Could you check a few things on this model? Use its own coordinates, in mm. A direction names the side the tool comes from. Coordinates: 2 decimals unless noted, no trailing zeros. Loops run counter-clockwise (first coordinate to the right, second up) from the corner with the lowest first, then second, coordinate; pieces in that order, holes last. Notation, with made-up numbers: (14, 10) - (37, 10) arc R15 ccw to (37, 39) - close; hole circle Ø3 at (-21, 8). An arc over 180 degrees is marked (long way). One line per question, with ' | ' between items. Start each with the question number.
1. I want a section at D-D, the plane x = 22.5. Write out the boundary of the cut face in (y, z), then the cut area to 3 significant figures.
2. Which directions (+Z, -Z, +X, -X, +Y, -Y) give clear straight access to the entire face, cutting with the end or side of a thin tool? Please do faces 1 (the flat face through (-10, 0, 2)), 2 (the flat face through (60, 14, 1)), 3 (the flat face through (0, 7, 1)), 4 (the cylindrical face through (45.9, 71.64, 1.48)).
3. I'm going to push flat-ended pins straight in: P1, Ø10, axis at x = 36, y = 87.5, coming from the -Z side; P2, Ø3.5, axis at x = -10.5, z = 2, coming from the +Y side; P3, Ø4, axis at x = 43, z = 10, coming from the +Y side; P4, Ø1.5, axis at x = -29, y = 18.5, coming from the +Z side. Where does each tip first touch, or does it pass through?
4. I want a section at A-A, the plane z = 9.5. Count the separate pieces of the cut face and the enclosed holes in it, then the cut area to 3 significant figures.
5. I want a section at C-C, the plane y = 90. Write out the boundary of the cut face in (x, z), then the cut area to 3 significant figures.
6. We'd pull the mould along X, two halves only. Please class faces 5 (the cylindrical face through (0.86, 109.1, 1.52)), 6 (the flat face through (-31, 19, 18)), 7 (the cylindrical face through (-30.8, 20.27, 10.4)): pulls with the +X half, pulls with the -X half, needs draft (parallel to the pull), parting line crosses it, or undercut.
7. I want a section at B-B, the plane x = -10. Write out the boundary of the cut face in (y, z).
8. Please list where these lines run through material, in increasing order: L1, parallel to Y at x = -17, z = 3.6; L2, parallel to X at y = 101, z = 8.25; L3, parallel to X at y = 90, z = 1.3. Write a range as [from, to].
from build123d import *

# Parameters (mm, degrees)
SKETCH_1_W          = 60
SKETCH_1_H          = 100
EXTRUDE_1_DEPTH     = 3
CUT_EXTRUDE_1_REACH = 118.658
SKETCH_2_R          = 1.6
SKETCH_3_W          = 100
SKETCH_3_H          = 25
EXTRUDE_2_DEPTH     = 3
SKETCH_4_R          = 2.5
EXTRUDE_3_DEPTH     = 3
SKETCH_5_R          = 1
CUT_EXTRUDE_2_DEPTH = 129.202964084
SKETCH_6_W          = 45
SKETCH_6_H          = 5
EXTRUDE_4_DEPTH     = 5
SKETCH_7_W          = 75
SKETCH_7_H          = 5
EXTRUDE_5_DEPTH     = 5
SKETCH_8_R          = 0.6
CUT_EXTRUDE_3_DEPTH = 5
SKETCH_9_W          = 35
SKETCH_9_H          = 73
EXTRUDE_6_DEPTH     = 3
SKETCH_10_R         = 2.5
EXTRUDE_7_DEPTH     = 15
SKETCH_11_R         = 1.5
CUT_EXTRUDE_4_DEPTH = 10
SKETCH_12_W         = 60
SKETCH_12_H         = 10
EXTRUDE_8_DEPTH     = 28
CUT_EXTRUDE_5_REACH = 153.026
CUT_EXTRUDE_6_REACH = 160.458
SKETCH_14_R         = 1.5
CUT_EXTRUDE_7_REACH = 139.335
SKETCH_15_W         = 50
SKETCH_15_H         = 45
SKETCH_15_W_2       = 15
FILLET_1_R          = 3
FILLET_2_R          = 3
FILLET_3_R          = 3
FILLET_4_R          = 3
FILLET_5_R          = 3
FILLET_6_R          = 3


with BuildPart() as part:
    # 草图1 → 凸台-拉伸1 (new body)
    with BuildSketch(Plane.XY):
        with Locations((30, 50)):
            Rectangle(SKETCH_1_W, SKETCH_1_H)
    extrude(amount=EXTRUDE_1_DEPTH)

    # 草图2 → 切除-拉伸1 (cut, up to next)
    with BuildSketch(Plane.XY.offset(3), mode=Mode.PRIVATE) as cut_extrude_1_sk1:
        with Locations((7.5, 90)):
            Circle(SKETCH_2_R)
    cut_extrude_1_tool1 = extrude(cut_extrude_1_sk1.sketch, amount=-CUT_EXTRUDE_1_REACH, mode=Mode.PRIVATE) & part.part
    # 草图2 → 切除-拉伸1 (cut, up to next)
    with BuildSketch(Plane.XY.offset(3), mode=Mode.PRIVATE) as cut_extrude_1_sk2:
        with Locations((52.5, 90)):
            Circle(SKETCH_2_R)
    cut_extrude_1_tool2 = extrude(cut_extrude_1_sk2.sketch, amount=-CUT_EXTRUDE_1_REACH, mode=Mode.PRIVATE) & part.part
    # 草图2 → 切除-拉伸1 (cut, up to next)
    with BuildSketch(Plane.XY.offset(3), mode=Mode.PRIVATE) as cut_extrude_1_sk3:
        with Locations((52.5, 20)):
            Circle(SKETCH_2_R)
    cut_extrude_1_tool3 = extrude(cut_extrude_1_sk3.sketch, amount=-CUT_EXTRUDE_1_REACH, mode=Mode.PRIVATE) & part.part
    # 草图2 → 切除-拉伸1 (cut, up to next)
    with BuildSketch(Plane.XY.offset(3), mode=Mode.PRIVATE) as cut_extrude_1_sk4:
        with Locations((7.5, 20)):
            Circle(SKETCH_2_R)
    cut_extrude_1_tool4 = extrude(cut_extrude_1_sk4.sketch, amount=-CUT_EXTRUDE_1_REACH, mode=Mode.PRIVATE) & part.part
    add(cut_extrude_1_tool1.solids().sort_by_distance((7.5, 90, 3))[0], mode=Mode.SUBTRACT)
    add(cut_extrude_1_tool2.solids().sort_by_distance((52.5, 90, 3))[0], mode=Mode.SUBTRACT)
    add(cut_extrude_1_tool3.solids().sort_by_distance((52.5, 20, 3))[0], mode=Mode.SUBTRACT)
    add(cut_extrude_1_tool4.solids().sort_by_distance((7.5, 20, 3))[0], mode=Mode.SUBTRACT)

    # 草图3 → 凸台-拉伸2 (add)
    with BuildSketch(Plane.XY.offset(3)):
        with Locations((30, -12.5)):
            Rectangle(SKETCH_3_W, SKETCH_3_H)
    extrude(amount=-EXTRUDE_2_DEPTH)

    # 草图4 → 凸台-拉伸3 (add)
    with BuildSketch(Plane.XY.offset(3)):
        with Locations(Location((-17, -3.5, 0), (0, 0, 180))):
            Circle(SKETCH_4_R)
        with Locations(Location((-17, -21.5, 0), (0, 0, 180))):
            Circle(SKETCH_4_R)
        with Locations(Location((77, -21.5, 0), (0, 0, 180))):
            Circle(SKETCH_4_R)
        with Locations(Location((77, -3.5, 0), (0, 0, 180))):
            Circle(SKETCH_4_R)
    extrude(amount=EXTRUDE_3_DEPTH)

    # 草图5 → 切除-拉伸2 (cut, through all)
    with BuildSketch(Plane.XY.offset(6)):
        with Locations((-17, -3.5)):
            Circle(SKETCH_5_R)
        with Locations((-17, -21.5)):
            Circle(SKETCH_5_R)
        with Locations((77, -21.5)):
            Circle(SKETCH_5_R)
        with Locations((77, -3.5)):
            Circle(SKETCH_5_R)
    extrude(amount=-CUT_EXTRUDE_2_DEPTH, mode=Mode.SUBTRACT)

    # 草图6 → 凸台-拉伸4 (add)
    with BuildSketch(Plane.XY.offset(3)):
        with Locations((30, 7.5)):
            Rectangle(SKETCH_6_W, SKETCH_6_H)
    extrude(amount=EXTRUDE_4_DEPTH)

    # 草图7 → 凸台-拉伸5 (add)
    with BuildSketch(Plane.XY.offset(8)):
        with Locations((30, 7.5)):
            Rectangle(SKETCH_7_W, SKETCH_7_H)
    extrude(amount=EXTRUDE_5_DEPTH)

    # 草图8 → 切除-拉伸3 (cut)
    with BuildSketch(Plane.XY.offset(13)):
        with Locations((-5, 7.5)):
            Circle(SKETCH_8_R)
        with Locations((30, 7.5)):
            Circle(SKETCH_8_R)
        with Locations((65, 7.5)):
            Circle(SKETCH_8_R)
    extrude(amount=-CUT_EXTRUDE_3_DEPTH, mode=Mode.SUBTRACT)

    # 草图9 → 凸台-拉伸6 (add)
    with BuildSketch(Plane.XY.offset(3)):
        with Locations((-17.5, 50)):
            Rectangle(SKETCH_9_W, SKETCH_9_H)
    extrude(amount=-EXTRUDE_6_DEPTH)

    # 草图10 → 凸台-拉伸7 (add)
    with BuildSketch(Plane.XY.offset(3)):
        with Locations(Location((-29.65, 81.95, 0), (0, 0, 180))):
            Circle(SKETCH_10_R)
        with Locations(Location((-5.35, 81.95, 0), (0, 0, 180))):
            Circle(SKETCH_10_R)
        with Locations(Location((-5.35, 18.05, 0), (0, 0, 180))):
            Circle(SKETCH_10_R)
        with Locations(Location((-29.65, 18.05, 0), (0, 0, 180))):
            Circle(SKETCH_10_R)
    extrude(amount=EXTRUDE_7_DEPTH)

    # 草图11 → 切除-拉伸4 (cut)
    with BuildSketch(Plane.XY.offset(18)):
        with Locations((-29.65, 81.95)):
            Circle(SKETCH_11_R)
        with Locations((-5.35, 81.95)):
            Circle(SKETCH_11_R)
        with Locations((-5.35, 18.05)):
            Circle(SKETCH_11_R)
        with Locations((-29.65, 18.05)):
            Circle(SKETCH_11_R)
    extrude(amount=-CUT_EXTRUDE_4_DEPTH, mode=Mode.SUBTRACT)

    # 草图12 → 凸台-拉伸8 (add)
    with BuildSketch(Plane(origin=(0, 0, 0), x_dir=(-1, 0, 0), z_dir=(0, 0, -1))):
        with Locations((-30, 105)):
            Rectangle(SKETCH_12_W, SKETCH_12_H)
    extrude(amount=-EXTRUDE_8_DEPTH)

    # 草图13 → 切除-拉伸5 (cut, up to next)
    with BuildSketch(Plane.XZ.offset(-100), mode=Mode.PRIVATE) as cut_extrude_5_sk1:
        with BuildLine():
            Line((3.5, 3), (3.5, 18))
            ThreePointArc((3.5, 18), (7.5, 22), (11.5, 18))
            Line((11.5, 18), (11.5, 3))
            Line((11.5, 3), (48.5, 3))
            Line((48.5, 3), (48.5, 18))
            ThreePointArc((48.5, 18), (52.5, 22), (56.5, 18))
            Line((56.5, 18), (56.5, 3))
            Line((56.5, 3), (60, 3))
            Line((60, 3), (60, 28))
            Line((60, 28), (0, 28))
            Line((0, 28), (0, 3))
            Line((0, 3), (3.5, 3))
        make_face()
    cut_extrude_5_tool1 = extrude(cut_extrude_5_sk1.sketch, amount=-CUT_EXTRUDE_5_REACH, mode=Mode.PRIVATE) & part.part
    add(cut_extrude_5_tool1.solids().sort_by_distance((30, 100, 16.317537))[0], mode=Mode.SUBTRACT)

    # 草图14 → 切除-拉伸6 (cut, up to next)
    with BuildSketch(Plane(origin=(0, 110, 0), x_dir=(1, 0, 0), z_dir=(0, 1, 0)), mode=Mode.PRIVATE) as cut_extrude_6_sk1:
        with Locations(Location((7.5, -18, 0), (0, 0, 180))):
            Circle(SKETCH_14_R)
    cut_extrude_6_tool1 = extrude(cut_extrude_6_sk1.sketch, amount=-CUT_EXTRUDE_6_REACH, mode=Mode.PRIVATE) & part.part
    # 草图14 → 切除-拉伸6 (cut, up to next)
    with BuildSketch(Plane(origin=(0, 110, 0), x_dir=(1, 0, 0), z_dir=(0, 1, 0)), mode=Mode.PRIVATE) as cut_extrude_6_sk2:
        with Locations(Location((52.5, -18, 0), (0, 0, 180))):
            Circle(SKETCH_14_R)
    cut_extrude_6_tool2 = extrude(cut_extrude_6_sk2.sketch, amount=-CUT_EXTRUDE_6_REACH, mode=Mode.PRIVATE) & part.part
    add(cut_extrude_6_tool1.solids().sort_by_distance((7.5, 110, 18))[0], mode=Mode.SUBTRACT)
    add(cut_extrude_6_tool2.solids().sort_by_distance((52.5, 110, 18))[0], mode=Mode.SUBTRACT)

    # 草图15 → 切除-拉伸7 (cut, up to next)
    with BuildSketch(Plane.XY.offset(3), mode=Mode.PRIVATE) as cut_extrude_7_sk1:
        with Locations((-10, 50)):
            Rectangle(SKETCH_15_W, SKETCH_15_H)
    cut_extrude_7_tool1 = extrude(cut_extrude_7_sk1.sketch, amount=-CUT_EXTRUDE_7_REACH, mode=Mode.PRIVATE) & part.part
    # 草图15 → 切除-拉伸7 (cut, up to next)
    with BuildSketch(Plane.XY.offset(3), mode=Mode.PRIVATE) as cut_extrude_7_sk2:
        with Locations((52.5, 50)):
            Rectangle(SKETCH_15_W_2, SKETCH_15_H)
    cut_extrude_7_tool2 = extrude(cut_extrude_7_sk2.sketch, amount=-CUT_EXTRUDE_7_REACH, mode=Mode.PRIVATE) & part.part
    add(cut_extrude_7_tool1.solids().sort_by_distance((-10, 50, 3))[0], mode=Mode.SUBTRACT)
    add(cut_extrude_7_tool2.solids().sort_by_distance((52.5, 50, 3))[0], mode=Mode.SUBTRACT)

    # 圆角1
    fillet_1_edges = [part.edges().sort_by_distance(p)[0] for p in [
        (15, 27.5, 1.5),
    ]]
    fillet(fillet_1_edges, radius=FILLET_1_R)

    # 圆角2
    fillet_2_edges = [part.edges().sort_by_distance(p)[0] for p in [
        (15, 72.5, 1.5),
    ]]
    fillet(fillet_2_edges, radius=FILLET_2_R)

    # 圆角3
    fillet_3_edges = [part.edges().sort_by_distance(p)[0] for p in [
        (-35, 86.5, 1.5),
    ]]
    fillet(fillet_3_edges, radius=FILLET_3_R)

    # 圆角4
    fillet_4_edges = [part.edges().sort_by_distance(p)[0] for p in [
        (-35, 72.5, 1.5),
    ]]
    fillet(fillet_4_edges, radius=FILLET_4_R)

    # 圆角5
    fillet_5_edges = [part.edges().sort_by_distance(p)[0] for p in [
        (0, 110, 1.5),
    ]]
    fillet(fillet_5_edges, radius=FILLET_5_R)

    # 圆角6
    fillet_6_edges = [part.edges().sort_by_distance(p)[0] for p in [
        (-35, 13.5, 1.5),
        (0, 13.5, 1.5),
        (60, 110, 1.5),
        (-35, 27.5, 1.5),
        (45, 72.5, 1.5),
        (60, 72.5, 1.5),
        (60, 27.5, 1.5),
        (45, 27.5, 1.5),
        (-20, -25, 1.5),
        (-20, 0, 1.5),
        (80, 0, 1.5),
        (80, -25, 1.5),
        (60, 0, 1.5),
        (0, 0, 1.5),
    ]]
    fillet(fillet_6_edges, radius=FILLET_6_R)


solid = part.part
Results are:
1) outline: (-25, 0) - (110, 0) - (110, 3) - (10, 3) - (10, 13) - (5, 13) - (5, 3) - (-25, 3) - close | area: 455 mm2
2) face 1: +Z, -Z, -X | face 2: -Z, +X, +Y | face 3: -Z, -X | face 4: +Z, -Z, +X
3) P1: stops at z = 0 | P2: stops at y = 86.5 | P3: stops at y = 10 | P4: stops at z = 18
4) separate pieces: 7 | enclosed holes: 7 | area: 582 mm2
5) outline: (0, 0) - (5.9, 0) - (5.9, 3) - (0, 3) - close; (9.1, 0) - (50.9, 0) - (50.9, 3) - (9.1, 3) - close; (54.1, 0) - (60, 0) - (60, 3) - (54.1, 3) - close | area: 161 mm2
6) face 5: pulls with the -X half | face 6: needs draft | face 7: undercut
7) outline: (-25, 0) - (0, 0) - (0, 3) - (-25, 3) - close; (13.5, 0) - (27.5, 0) - (27.5, 3) - (13.5, 3) - close; (72.5, 0) - (86.5, 0) - (86.5, 3) - (72.5, 3) - close
8) L1: y = [-24, -22.5], [-20.5, -19], [-6, -4.5], [-2.5, -1] | L2: x = [3.5, 11.5], [48.5, 56.5] | L3: x = [0, 5.9], [9.1, 50.9], [54.1, 60]
